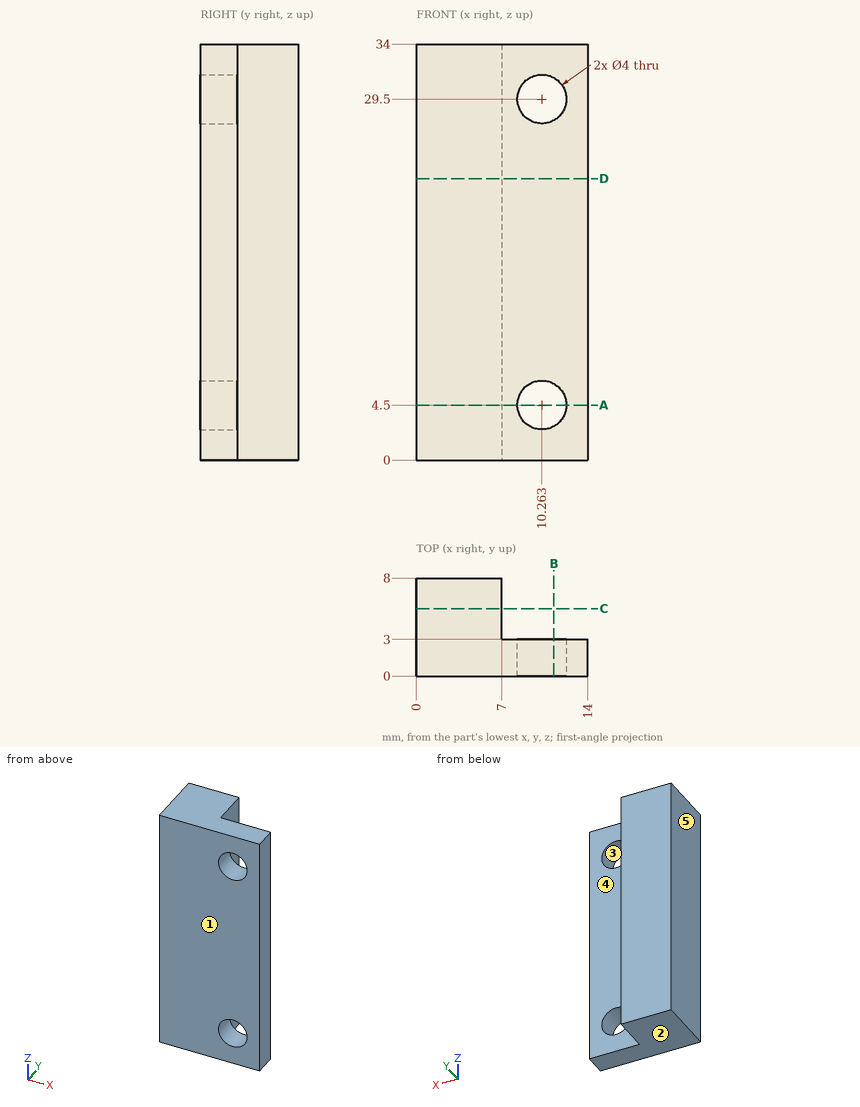
Could you check a few things on this drawing? It's one solid part, dimensions in mm from its lowest x, y, z. A direction names the side the tool comes from. Round coordinates to 2 decimals unless told otherwise and drop trailing zeros. Order: outer loops, then holes, each group sorted by start corner. A loop starts at its lowest first (then second) coordinate and runs counter-clockwise, first axis right, second up.
Q1. Imagine slicing it at D-D, the plane z = 23. List the corners of the cut face in (x, y) for me.
Geometry says:
outline: (0, 0) - (14, 0) - (14, 3) - (7, 3) - (7, 8) - (0, 8) - close
Q2. Imagine slicing it at A-A, the plane z = 4.5. List the corners of the cut face in (x, y) for me, then the cut area to 3 significant figures.
Geometry says:
outline: (0, 0) - (8.26, 0) - (8.26, 3) - (7, 3) - (7, 8) - (0, 8) - close; (12.26, 0) - (14, 0) - (14, 3) - (12.26, 3) - close
area: 65.0 mm2
Q3. Which directions (+Z, -Z, +X, -X, +Y, -Y) give clear straight access to the entire face, cutting with the end or side of a thin tool? Please do the marked faces 4 and 5.
Geometry says:
face 4: +Z, -Z, +X, +Y
face 5: +Z, -Z, -X, +Y, -Y
Q4. Imagine slicing it at C-C, the plane y = 5.5. List the corners of the cut face in (x, z) for me.
Geometry says:
outline: (0, 0) - (7, 0) - (7, 34) - (0, 34) - close
Q5. I'm going to push flat-ended pins straight in: P1, Ø5.5, axis at x = 12, z = 21, coming from the +Y side; P2, Ø2.5, axis at x = 10.26, z = 4.5, coming from the -Y side; P3, Ø1.5, axis at y = 6.5, z = 22.5, coming from the +X side. Where does each tip first touch, or does it pass through?
Geometry says:
P1: stops at y = 3
P2: passes through
P3: stops at x = 7
Q6. Thinking about a two-plate mould opening in Z: for the marked faces 1, 2 and 3, which applies, released by +Z, released by -Z, zero draft, split by the parting line, or undercut?
Geometry says:
face 1: zero draft
face 2: released by -Z
face 3: undercut
Q7. Imagine slicing it at B-B, the plane x = 11.25. List the corners of the cut face in (y, z) for me.
Geometry says:
outline: (0, 0) - (3, 0) - (3, 2.76) - (0, 2.76) - close; (0, 6.24) - (3, 6.24) - (3, 27.76) - (0, 27.76) - close; (0, 31.24) - (3, 31.24) - (3, 34) - (0, 34) - close
Q8. Please list where these lines run through material, in increasing order: probe 1 along X at (y, z) = (2, 29.5); probe 2 along Y at (x, z) = (10.25, 16); probe 3 along X at (y, z) = (5.5, 13.5).
Geometry says:
probe 1: x = 0 to 8.26, 12.26 to 14
probe 2: y = 0 to 3
probe 3: x = 0 to 7
